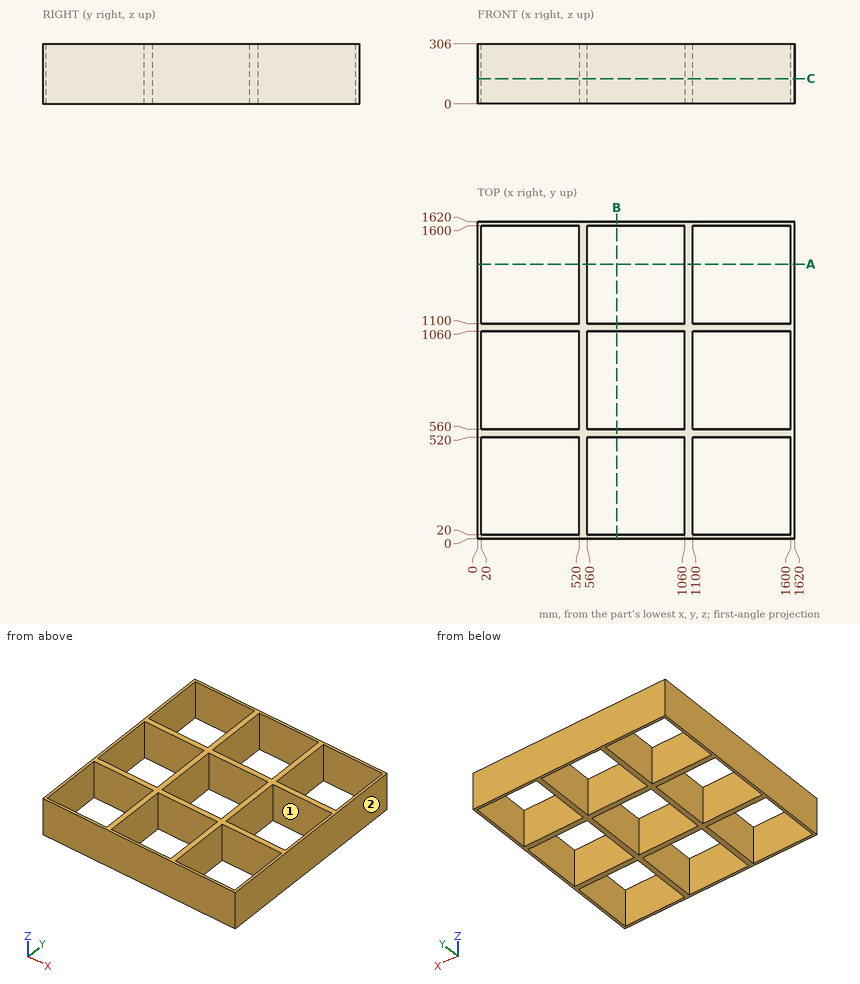
For this review, use the dimensioned drawing (mm, ordinates from the lowest corner) and the shaded views. Round coordinates to 2 decimals unless told otherwise and drop trailing zeros. Order: outer loops, then holes, each group sorted by start corner. A loop starts at its lowest first (then second) coordinate and runs counter-clockwise, first axis right, second up. Notation, with made-up numbers: (-19.5, -32.5) -> (-12.5, -32.5) arc R10 ccw to (-12.5, -17.5) -> close; hole circle Ø2 at (31, 21.25). An arc over 180 degrees is marked (long way). Write item = value, one per line. Start each with the question number.
Item 1: Consider section A-A on y = 1404.5. Write out the cut boundary in (x, z).
Item 2: Consider section C-C on z = 128.5. Count the separate pieces of the cut face and the enclosed holes in it, plus the area to 3 significant figures.
Item 3: For line 1 along Y through (x, z) = (1241, 104), list the stretches that pass through material, from the lowest coordinate up.
Item 4: Mouldability with a two-part tool opening along X and no side actions: class the marked faces 1 and 2 as released by +X, released by -X, zero draft, split by the parting line, or undercut.
Item 5: Clearance check with a flat-ended pin moving along its axis: pin 1 Ø12 at (x, z) = (304.5, 215) entering from -Y. State where the tip first meets the part, or that it passes through.
Conclusion:
q1.outline = (0, 0) -> (20, 0) -> (20, 306) -> (0, 306) -> close; (520, 0) -> (560, 0) -> (560, 306) -> (520, 306) -> close; (1060, 0) -> (1100, 0) -> (1100, 306) -> (1060, 306) -> close; (1600, 0) -> (1620, 0) -> (1620, 306) -> (1600, 306) -> close
q2.separate_pieces = 1
q2.enclosed_holes = 9
q2.area = 374,000 mm2
q3.line_1 = 0 to 20, 520 to 560, 1060 to 1100, 1600 to 1620
q4.face_1 = undercut
q4.face_2 = released by +X
q5.pin_1 = 0
